Could you check a few things on this drawing? It's one solid part, dimensions in mm from its lowest x, y, z. Give positions to 0.01 mm unless a question says otherwise; leave off trailing zeros. Write each loop counter-clockwise with the first axis right and the second up, starting at its lowest first coordinate (ties: lowest second). Pieces come first, ordered by that corner, then holes. Notation, with made-up numbers: (26.25, 38.5) -> (69.25, 38.5) arc R30 ccw to (69.25, 63.5) -> close; hole circle Ø4 at (88.25, -38). An arc over 180 degrees is marked (long way). Use CSV: the item, a comma, the result in double quotes. Start each with the question number.
(1) If we mould it in two halves opening along X, with no side actions, what happens to the marked faces 1 and 2? For each: pulls with the +X half, pulls with the -X half, needs draft (parallel to the pull), parting line crosses it, or undercut.
(2) Suppose I cut it at A-A on y = 112.5. List the corners of the cut face in (x, z) for me, plus the area to 3 significant figures.
(3) Suppose I cut it at C-C on x = 60. List the corners of the cut face in (y, z) for me.
(4) Suppose I cut it at B-B on z = 3.75. List the corners of the cut face in (x, y) for me.
(5) I need wall thicknesses on L1, parallel to X at y = 114, z = 8.75; L2, parallel to X at y = 18, z = 8.25; L3, parallel to Y at x = 51, z = 3.25. Which ranges of each line are inside material? Lowest first, please. Write a range as [from, to].
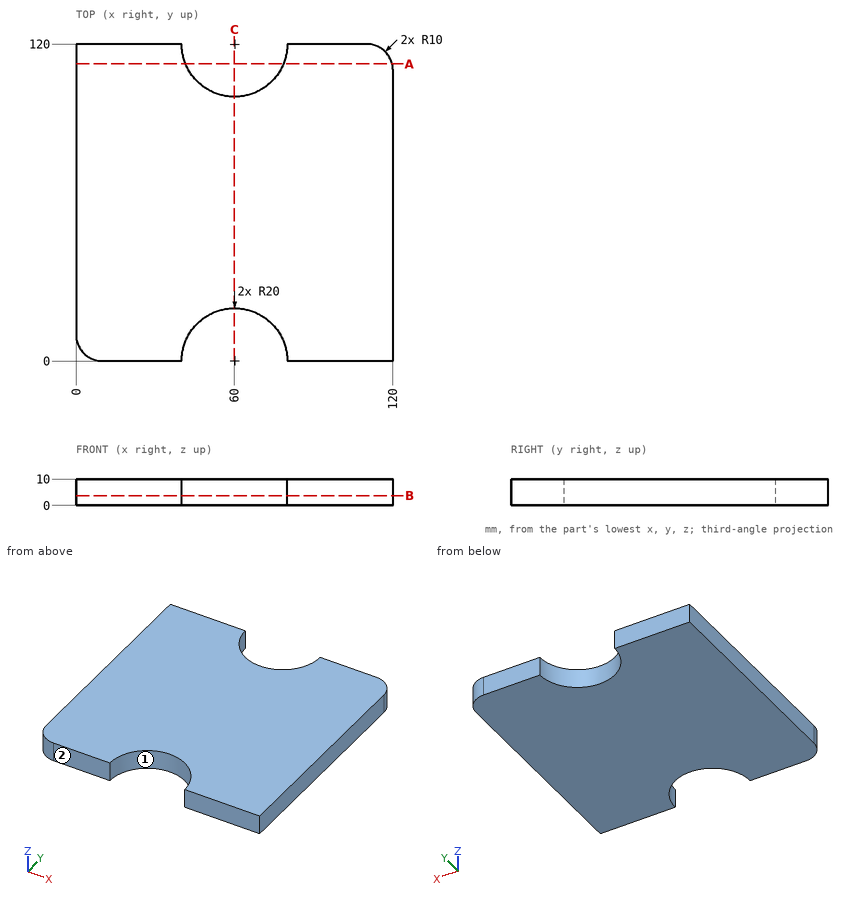
Geometry says:
1,face 1,"undercut"
1,face 2,"needs draft"
2,outline,"(0, 0) -> (41.46, 0) -> (41.46, 10) -> (0, 10) -> close; (78.54, 0) -> (119.68, 0) -> (119.68, 10) -> (78.54, 10) -> close"
2,area,"826 mm²"
3,outline,"(20, 0) -> (100, 0) -> (100, 10) -> (20, 10) -> close"
4,outline,"(0, 10) arc R10 ccw to (10, 0) -> (40, 0) arc R20 cw to (80, 0) -> (120, 0) -> (120, 110) arc R10 ccw to (110, 120) -> (80, 120) arc R20 cw to (40, 120) -> (0, 120) -> close"
5,L1,"[0, 40.92], [79.08, 119.17]"
5,L2,"[0, 51.28], [68.72, 120]"
5,L3,"[17.86, 102.14]"
